from build123d import *

# Parameters (mm, degrees)
F0_R     = 5.08
F1_DEPTH = 8.89
F0_R_2   = 6.985
F2_DEPTH = 3.81
F3_R     = 0.6604


with BuildPart() as f1:
    # F0 (on Top) → F1 (new body)
    with BuildSketch(Plane.XY):
        Circle(F0_R)
    extrude(amount=F1_DEPTH)

    # F0 (on Top) → F2 (join)
    with BuildSketch(Plane.XY):
        Circle(F0_R_2)
        Circle(F0_R, mode=Mode.SUBTRACT)
    extrude(amount=F2_DEPTH)

    # F3
    f3_edges = [f1.edges().sort_by_distance(p)[0] for p in [
        (-6.985, 0, 3.81),
        (-5.08, 0, 3.81),
    ]]
    fillet(f3_edges, radius=F3_R)


solid = f1.part
Here's how the part is built. I have some questions about the finished solid (model axes, mm). A direction names the side the tool comes from. Coordinates: 2 decimals unless noted, no trailing zeros. Order: outer loops, then holes, each group sorted by start corner. A loop starts at its lowest first (then second) coordinate and runs counter-clockwise, first axis right, second up. Notation, with made-up numbers: (46.5, 4) - (62.5, 4) arc R15 ccw to (62.5, 14) - close; hole circle Ø9 at (78.5, -25). An arc over 180 degrees is marked (long way). Use CSV: the item, a comma, the result in double quotes. Start each with the question number.
1. If we mould it in two halves opening along X, with no side actions, what happens to faces 3 (the face through (-0.909, 6.926, 1.553)), 4 (the face through (0, 0, 8.89))? For each: +X half, -X half, draft (parallel to the pull), parting line (faces both ways), or undercut.
2. Please list where these lines run through material, in increasing order: line 1 (Z direction, x = -6, y = 2); line 2 (Y direction, x = -3, z = 6); line 3 (Y direction, x = 5, z = 1.5). Write a range as from..to.
3. Suppose I cut it at A-A on y = 0. List the corners of the cut face in (x, z) for me (3 decimals).
4. Suppose I cut it at D-D on z = 2.5. List the corners of the cut face in (x, y) for me (3 decimals).
5. Suppose I cut it at C-C on z = 8. List the corners of the cut face in (x, y) for me.
6. I'm going to push flat-ended pins straight in: pin 1 (5 mm diameter, centred on y = -4.5, z = 6.5, fed in from -X); pin 2 (2 mm diameter, centred on x = 0.5, z = 7, fed in from +Y); pin 3 (1.5 mm diameter, centred on y = -0.5, z = 5, fed in from +X). Where does each tip first touch, or does it pass through?
7. For faces 1 (the face through (0, 0, 0)), 2 (the face through (1, -6, 3.81)), which set-ups out of +Z, -Z, +X, -X, +Y, -Y let a thin tool reach every point of the face, with its end or its side?
Output:
1,face 3,"parting line"
1,face 4,"draft"
2,line 1,"z = 0..3.81"
2,line 2,"y = -4.1..4.1"
2,line 3,"y = -4.88..4.88"
3,outline,"(-6.985, 0) - (6.985, 0) - (6.985, 3.15) arc R0.66 ccw to (6.325, 3.81) - (5.74, 3.81) arc R0.66 cw to (5.08, 4.47) - (5.08, 8.89) - (-5.08, 8.89) - (-5.08, 4.47) arc R0.66 cw to (-5.74, 3.81) - (-6.325, 3.81) arc R0.66 ccw to (-6.985, 3.15) - close"
4,outline,"circle Ø13.97 at (0, 0)"
5,outline,"circle Ø10.16 at (0, 0)"
6,pin 1,"stops at x = -4.67"
6,pin 2,"stops at y = 5.08"
6,pin 3,"stops at x = 5.1"
7,face 1,"-Z, +X, -X, +Y, -Y"
7,face 2,"+Z"
